Autodesk Inventor part; units mm, degrees
ref_plane "YZ Plane" through (0, 0, 0) normal (1, 0, 0) x (0, 1, 0)
ref_plane "XZ Plane" through (0, 0, 0) normal (0, 1, 0) x (-1, 0, 0)
ref_plane "XY Plane" through (0, 0, 0) normal (0, 0, 1) x (1, 0, 0)
sketch "Sketch1" plane through (0, 0, 0) normal (0, 0, 1) x (1, 0, 0)
  circle A0 centre (0, 0) radius 25.7048
  dimension "d0" = 51.4096
extrude "Extrusion1" add sketch "Sketch1" along normal blind 6.4262
sketch "Sketch2" plane through (0, 0, 6.4262) normal (0, 0, 1) x (1, 0, 0)
  circle A0 centre (0, 0) radius 8.0645
  dimension "d3" = 16.129
extrude "Extrusion2" cut sketch "Sketch2" against normal blind 127
sketch "Sketch3" plane through (0, 0, 0) normal (0, 0, -1) x (-1, 0, 0)
  circle A0 centre (0, 0) radius 29.9085
  dimension "d6" = 59.817
extrude "Extrusion3" add sketch "Sketch3" along normal blind 3.2512
sketch "Sketch4" plane through (0, 0, 6.4262) normal (0, 0, 1) x (1, 0, 0)
  circle A0 centre (0, 0) radius 8.0645
extrude "Extrusion4" cut sketch "Sketch4" against normal blind 127
sketch "Sketch5" plane through (0, 0, -3.2512) normal (0, 0, -1) x (-1, 0, 0)
  circle A0 centre (23.7744, 0) radius 2.6416
  circle A1 centre (-23.7744, 0) radius 2.6416
  circle A2 centre (0, 0) radius 29.9085
  circle A3 centre (0, 0) radius 8.0645
  line L0 (0, 8.0645) -> (0, -8.0645) construction
  dimension "d11" = 5.2832
  dimension "d12" = 42.2656
extrude "Extrusion5" cut sketch "Sketch5" against normal through all contours A0 | A1
pattern_circular "Circular Pattern1" count 3 over 360 about axis through (0, 0, 6.4262) along (0, 0, -1) of "Extrusion5"
CAD build for the part. Positions are in the model's coordinates, mm. A direction names the side the tool comes from. Round coordinates to 2 decimals unless told otherwise and drop trailing zeros. Write each loop counter-clockwise with the first axis right and the second up, starting at its lowest first coordinate (ties: lowest second). Pieces come first, ordered by that corner, then holes. Notation, with made-up numbers: M 8,58 L 15,58 A20 cw 15,72 Z; hole C -5,83.25 d7. An arc over 180 degrees is marked long. Use a Markdown table: item, result. Add a question column.
1. 3-axis set-ups, long thin cutter, end or side, ignore diameter. For faces 4 (the face through (-22.342, 12.712, 3.168)), 5 (the face through (22.18, 12.99, 3.17)), 6 (the face through (25, -9, 0)), 7 (the face through (-22.18, -12.99, 3.17)): which of +Z, -Z, +X, -X, +Y, -Y reach the whole face in a straight line?
2. Pull direction X, two halves, no side cores. Call faces 1 (the face through (-6, 6, 6.426)), 2 (the face through (22.342, -12.712, 3.168)), 3 (the face through (-11.31, 18.01, 1.52)): released by +X, released by -X, zero draft, split by the parting line, or undercut.
3. Slice it at D-D on y = 22. Give the cut face in (x, z), then the cut area to 3 significant figures.
4. Flat gauge pins, fed straight in: P1, Ø3, axis at x = 5, z = -0.5, coming from the +Y side; P2, Ø3, axis at x = 11.89, y = 20.59, coming from the -Z side; P3, Ø2, axis at y = -7, z = 5, coming from the -X side; P4, Ø2, axis at y = 13.5, z = 0.5, coming from the -X side. Where does each tip first touch, or does it go through?
5. Slice it at A-A on y = 0. Give the cut face in (x, z), then the cut area to 3 significant figures.
6. Drill centre lines: probe 1 along Y at (x, z) = (0, -0.5); probe 2 along Z at (x, y) = (-17.5, 21); probe 3 along Y at (x, z) = (12, 1.25). Where is each one in solid material? Low to high.
7. Slice it at C-C on z = 5. Give the cut face in (x, y).
8. Slice it at B-B on x = 0. Give the cut face in (y, z), then the cut area to 3 significant figures.
Reply:
| question | item | result |
|---|---|---|
| 1 | face 4 | +Z, -X, +Y |
| 1 | face 5 | +Z, +X, +Y |
| 1 | face 6 | +Z |
| 1 | face 7 | +Z, -X, -Y |
| 2 | face 1 | zero draft |
| 2 | face 2 | released by +X |
| 2 | face 3 | undercut |
| 3 | outline | M -20.26,-3.25 L -14.12,-3.25 L -14.12,0 L -20.26,0 Z; M -9.65,-3.25 L 9.65,-3.25 L 9.65,6.43 L -9.65,6.43 Z; M 14.12,-3.25 L 20.26,-3.25 L 20.26,0 L 14.12,0 Z |
| 3 | area | 227 mm^2 |
| 4 | P1 | stops at y = 29.7 |
| 4 | P2 | passes through |
| 4 | P3 | stops at x = -24.99 |
| 4 | P4 | stops at x = -27.11 |
| 5 | outline | M -29.91,-3.25 L -26.42,-3.25 L -26.42,0 L -29.91,0 Z; M -21.13,-3.25 L -8.06,-3.25 L -8.06,6.43 L -21.13,6.43 Z; M 8.06,-3.25 L 21.13,-3.25 L 21.13,6.43 L 8.06,6.43 Z; M 26.42,-3.25 L 29.91,-3.25 L 29.91,0 L 26.42,0 Z |
| 5 | area | 276 mm^2 |
| 6 | probe 1 | y = -29.91 to -8.06, 8.06 to 29.91 |
| 6 | probe 2 | z = -3.25 to 0 |
| 6 | probe 3 | y = -17.95 to 17.95 |
| 7 | outline | M -25.64,-1.87 A25.7 ccw -14.44,-21.26 A2.64 cw long -11.2,-23.14 A25.7 ccw 11.2,-23.14 A2.64 cw long 14.44,-21.26 A25.7 ccw 25.64,-1.87 A2.64 cw long 25.64,1.87 A25.7 ccw 14.44,21.26 A2.64 cw long 11.2,23.14 A25.7 ccw -11.2,23.14 A2.64 cw long -14.44,21.26 A25.7 ccw -25.64,1.87 A2.64 cw long Z; hole C 0,0 d16.13 |
| 8 | outline | M -29.91,-3.25 L -8.06,-3.25 L -8.06,6.43 L -25.7,6.43 L -25.7,0 L -29.91,0 Z; M 8.06,-3.25 L 29.91,-3.25 L 29.91,0 L 25.7,0 L 25.7,6.43 L 8.06,6.43 Z |
| 8 | area | 369 mm^2 |
